```python
from build123d import *

# Parameters (mm, degrees)
F0_W        = 250
F0_H        = 250
F0_R        = 15
F1_DEPTH    = 20
F2_R        = 5
F3_DEPTH    = 250
F5_T        = -2.5
F6_T1_DEPTH = 45
F6_T3_DEPTH = 275
F6_T5_DEPTH = 300


# Not quite as in the source:
# - a fillet or chamfer that OpenCascade refuses, or shapes differently, is made with other operations: its cross-section is extruded or revolved along the edge and cut away or added
# - the program builds the solid bodies; features that only make, move or delete a surface that nothing else refers to are left out


with BuildPart() as f1:
    # F0 (on Front) → F1 (new body)
    with BuildSketch(Plane.XZ):
        with Locations((79.7126553953, -72.3895989358)):
            Rectangle(F0_W, F0_H)
        with Locations((39.7126553953, -147.645547986)):
            Circle(F0_R, mode=Mode.SUBTRACT)
        with Locations((122.2126553953, -147.645547986)):
            Circle(F0_R, mode=Mode.SUBTRACT)
        with BuildLine():
            Line((-15.2873446047, -67.7264088296), (-15.2873446047, 18.6264493965))
            ThreePointArc((-15.2873446047, 18.6264493965), (-12.3539628579, 25.7082593932), (-5.2721528612, 28.64164114))
            Line((-5.2721528612, 28.64164114), (159.5934226625, 28.64164114))
            ThreePointArc((159.5934226625, 28.64164114), (170.2843346542, 24.2133203989), (174.7126553953, 13.5224084073))
            Line((174.7126553953, 13.5224084073), (174.7126553953, -67.7264088296))
            ThreePointArc((174.7126553953, -67.7264088296), (171.7792736485, -74.8082188263), (164.6974636518, -77.7416005731))
            Line((164.6974636518, -77.7416005731), (-5.2721528612, -77.7416005731))
            ThreePointArc((-5.2721528612, -77.7416005731), (-12.3539628579, -74.8082188263), (-15.2873446047, -67.7264088296))
        make_face(mode=Mode.SUBTRACT)
    extrude(amount=F1_DEPTH)

    # F2
    f2_edges = [f1.edges().sort_by_distance(p)[0] for p in [
        (204.712655, -10, 52.610401),
        (-45.287345, -10, 52.610401),
    ]]
    fillet(f2_edges, radius=F2_R)

    # F3 (add): a face of the model
    f3_faces = [f1.faces().sort_by_distance(p)[0] for p in [
        (79.7304888538, -20, -93.2584337022),
    ]]
    extrude(f3_faces, amount=F3_DEPTH)

    # F5
    f5_openings = [f1.faces().sort_by_distance(p)[0] for p in [
        (79.730489, -270, -93.258434),
    ]]
    offset(amount=F5_T, openings=f5_openings, kind=Kind.INTERSECTION)

    # F6: fillet of radius 10 on 5 edges, made by hand

    # F6_s2 → F6_t1 (cut)
    with BuildSketch(Plane.XZ.offset(-25)):
        with BuildLine():
            ThreePointArc((204.7126553953, -187.3895989358), (201.7837232071, -194.4606667477), (194.7126553953, -197.3895989358))
            Line((194.7126553953, -197.3895989358), (204.7126553953, -197.3895989358))
            Line((204.7126553953, -197.3895989358), (204.7126553953, -187.3895989358))
        make_face()
        with BuildLine():
            ThreePointArc((-35.2873446047, -197.3895989358), (-42.3584124166, -194.4606667477), (-45.2873446047, -187.3895989358))
            Line((-45.2873446047, -187.3895989358), (-45.2873446047, -197.3895989358))
            Line((-45.2873446047, -197.3895989358), (-35.2873446047, -197.3895989358))
        make_face()
    extrude(amount=F6_T1_DEPTH, mode=Mode.SUBTRACT)

    # F6_s4 → F6_t3 (cut)
    with BuildSketch(Plane.XZ.offset(20)):
        with BuildLine():
            ThreePointArc((204.7126553953, -187.3895989358), (201.7837232071, -194.4606667477), (194.7126553953, -197.3895989358))
            Line((194.7126553953, -197.3895989358), (204.7126553953, -197.3895989358))
            Line((204.7126553953, -197.3895989358), (204.7126553953, -187.3895989358))
        make_face()
        with BuildLine():
            ThreePointArc((-35.2873446047, -197.3895989358), (-42.3584124166, -194.4606667477), (-45.2873446047, -187.3895989358))
            Line((-45.2873446047, -187.3895989358), (-45.2873446047, -197.3895989358))
            Line((-45.2873446047, -197.3895989358), (-35.2873446047, -197.3895989358))
        make_face()
    extrude(amount=F6_T3_DEPTH, mode=Mode.SUBTRACT)

    # F6_s6 → F6_t5 (cut)
    with BuildSketch(Plane.YZ.offset(-70.2873446047)):
        with BuildLine():
            ThreePointArc((-260, -197.3895989358), (-267.0710678119, -194.4606667477), (-270, -187.3895989358))
            Line((-270, -187.3895989358), (-270, -197.3895989358))
            Line((-270, -197.3895989358), (-260, -197.3895989358))
        make_face()
    extrude(amount=F6_T5_DEPTH, mode=Mode.SUBTRACT)


solid = f1.part
```
Can you work these out from the model? Positions are in its coordinate system, mm. A direction names the side the tool comes from. Give positions to 0.01 mm unless a question says otherwise; leave off trailing zeros. Order: outer loops, then holes, each group sorted by start corner. A loop starts at its lowest first (then second) coordinate and runs counter-clockwise, first axis right, second up. Notation, with made-up numbers: M 72.5,16 L 93.5,16 A29 ccw 93.5,54 Z; hole C -36,86.5 d11. An arc over 180 degrees is marked long. One line per item, written item: value.
1) I want a section at A-A, the plane x = 18. List the corners of the cut face in (y, z) for me, plus the area to 3 significant figures.
Answer sheet:
outline: M -270,-80.24 L -2.5,-80.24 L -2.5,-194.89 L -266.61,-194.89 A10 ccw -260,-197.39 L 0,-197.39 L 0,-77.74 L -270,-77.74 Z; M -270,28.64 L 0,28.64 L 0,52.61 L -270,52.61 L -270,50.11 L -2.5,50.11 L -2.5,31.14 L -270,31.14 Z
area: 3,020 mm^2
2) Please list where these lines run through material, in increasing order: line 1 along X through (y, z) = (-137.5, -30); line 2 along Z through (x, y) = (67.5, -62); line 3 along X through (y, z) = (-164, -165.5).
Answer sheet:
line 1: x = -45.29 to -42.79, -17.79 to -15.29, 174.71 to 177.21, 202.21 to 204.71
line 2: z = -197.39 to -194.89, -80.24 to -77.74, 28.64 to 31.14, 50.11 to 52.61
line 3: x = -45.29 to -42.79, 202.21 to 204.71
3) We'd pull the mould along Z, two halves only. Please class faces 1 (the face through (120.26, -133.11, -132.773)), 2 (the face through (53, -270, -140)), 3 (the face through (78, -134, 50.11)), 4 (the face through (-40.933, -133.11, -195.644)): released by +Z, released by -Z, zero draft, split by the parting line, or undercut.
Answer sheet:
face 1: undercut
face 2: zero draft
face 3: undercut
face 4: released by -Z
4) For P1, Ø1, axis at x = 123, z = -105, coming from the -Y side; P2, Ø10, axis at x = 52, z = -161.5, coming from the +Y side, each with a flat end and sliding along its axis, tell me the tip position at first contact or that it passes through.
Answer sheet:
P1: stops at y = -2.5
P2: stops at y = 0
5) I want a section at D-D, the plane x = 133. List the corners of the cut face in (y, z) for me, plus the area to 3 significant figures.
Answer sheet:
outline: M -270,-161.43 L -2.5,-161.43 L -2.5,-194.89 L -266.61,-194.89 A10 ccw -260,-197.39 L 0,-197.39 L 0,-158.07 L -270,-158.07 Z; M -270,-137.22 L 0,-137.22 L 0,-77.74 L -270,-77.74 L -270,-80.24 L -2.5,-80.24 L -2.5,-133.87 L -270,-133.87 Z; M -270,28.64 L 0,28.64 L 0,52.61 L -270,52.61 L -270,50.11 L -2.5,50.11 L -2.5,31.14 L -270,31.14 Z
area: 4,760 mm^2
6) I want a section at C-C, the plane z = -115. List the corners of the cut face in (x, y) for me.
Answer sheet:
outline: M -45.29,-270 L -42.79,-270 L -42.79,-2.5 L 202.21,-2.5 L 202.21,-270 L 204.71,-270 L 204.71,0 L -45.29,0 Z
7) On a 3-axis mill with a long thin cutter (end or side, diameter ignored), from which of +Z, -Z, +X, -X, +Y, -Y can I reach the whole of each face in a straight line? I mean faces 5 (the face through (37.4, -134.4, -130.3)), 6 (the face through (-12.276, -133.11, -74.886)), 7 (the face through (204.713, -133, -72)). Say none if no direction works.
Answer sheet:
face 5: -Y
face 6: +Y, -Y
face 7: +Z, -Z, +X, +Y, -Y
8) I want a section at B-B, the plane z = -5. List the corners of the cut face in (x, y) for me.
Answer sheet:
outline: M -45.29,-270 L -42.79,-270 L -42.79,-2.5 L -17.79,-2.5 L -17.79,-270 L -15.29,-270 L -15.29,0 L -45.29,0 Z; M 174.71,-270 L 177.21,-270 L 177.21,-2.5 L 202.21,-2.5 L 202.21,-270 L 204.71,-270 L 204.71,0 L 174.71,0 Z
